Autodesk Fusion 360 part; units mm, degrees
sketch "Sketch1" plane through (0, 0, 0) normal (0, 1, 0) x (1, 0, 0)
  circle A0 centre (0, 0) radius 7.9
  dimension "d1" = 15.8
extrude "Extrude1" add sketch "Sketch1" against normal blind 5.5
sketch "Sketch2" plane through (0, -5.5, 0) normal (0, -1, 0) x (1, 0, 0)
  circle A0 centre (0, 0) radius 7.9
  circle A1 centre (0, 0) radius 3.5
  dimension "d4" = 7
extrude "Extrude2" add sketch "Sketch2" along normal blind 2.7 contours A1
fillet "Fillet1" radius 1.5 1 edges at (-3.2631, -8.2, -1.2657)
extrude "Extrude3" add 1 faces at (3.1441, 0, -2.759) along direction (0, 1, 0) blind 1.3 draft -73.5
sketch "Sketch3" plane through (0, 1.3, 0) normal (0, 1, 0) x (-1, 0, 0)
  circle A0 centre (0, 0) radius 3.5113
  circle A1 centre (0, 0) radius 1.6
  line L0 (-1.02, 1.2327) -> (-1.02, -1.2327)
  dimension "d11" = 3.2
  dimension "d12" = 1.02
extrude "Extrude4" cut sketch "Sketch3" against normal blind 9.3 contours A1 L0 picked at (-0.3273, 0.4001)
sketch "Sketch4" plane through (0, 0, 0) normal (1, 0, 0) x (0, 1, 0)
  line L0 (1.3, 0) -> (1.3, -3.5113)
  line L1 (1.3, 3.5113) -> (1.3, 0)
  line L2 (-8.2, 0) -> (-8.2, 2)
  line L3 (-8.2, -2) -> (-8.2, 0)
  line L4 (-5.5, -3.5) -> (-5.5, -7.9)
  line L5 (-5.5, 7.9) -> (-5.5, 3.5)
  line L6 (1.3, 3.5113) -> (0, 7.9)
  line L7 (1.3, -3.5113) -> (0, -7.9)
  arc A0 (-8.2, -2) -> (-6.7, -3.5) centre (-6.7, -2) ccw
  arc A1 (-6.7, 3.5) -> (-8.2, 2) centre (-6.7, 2) ccw
  line L8 (-5.5, 3.5) -> (-6.7, 3.5)
  line L9 (-5.5, -3.5) -> (-6.7, -3.5)
  line L10 (0, 7.9) -> (-5.5, 7.9)
  line L11 (0, -7.9) -> (-5.5, -7.9)
  line L12 (-5.5, 7.9) -> (-5.5, -7.9)
  line L13 (0, -7.9) -> (0, 7.9)
  circle A2 centre (-2.75, 9.2007) radius 2.5
  point P0 (-4.885, 7.9)
  point P1 (-0.615, 7.9)
  dimension "d15" = 0.615
  dimension "d16" = 0.615
  dimension "d17" = 5
revolve "Revolve1" cut sketch "Sketch4" angle 360 about axis through (0, 1.75, 0) along (0, 1, 0) contours L10 A2 picked at (-2.75, 7.5002)
For this review, take the finished solid that the model builds, in its own axes (mm). A direction names the side the tool comes from. Coordinates: 2 decimals unless noted, no trailing zeros. Order: outer loops, then holes, each group sorted by start corner. A loop starts at its lowest first (then second) coordinate and runs counter-clockwise, first axis right, second up. Notation, with made-up numbers: (50.25, 78.25) -> (66.25, 78.25) arc R11 cw to (66.25, 88.25) -> close; hole circle Ø7 at (-21.5, 57.5). An arc over 180 degrees is marked (long way). Return JSON: item names as keys, results as strings.
1. We need section A-A on x = 0. Write out the cut boundary in (y, z), and give its area (3 significant figures).
Answer block:
{"outline": "(-8.2, -2) arc R1.5 ccw to (-6.7, -3.5) -> (-5.5, -3.5) -> (-5.5, -7.9) -> (-4.88, -7.9) arc R2.5 cw to (-0.62, -7.9) -> (0, -7.9) -> (1.3, -3.51) -> (1.3, -1.6) -> (-8, -1.6) -> (-8, 1.6) -> (1.3, 1.6) -> (1.3, 3.51) -> (0, 7.9) -> (-0.62, 7.9) arc R2.5 cw to (-4.88, 7.9) -> (-5.5, 7.9) -> (-5.5, 3.5) -> (-6.7, 3.5) arc R1.5 ccw to (-8.2, 2) -> close", "area": "82.7 mm²"}
2. We need section D-D on y = -2. Write out the cut boundary in (x, z).
Answer block:
{"outline": "circle Ø13.63 at (0, 0); hole (1.02, -1.23) -> (1.02, 1.23) arc R1.6 ccw (long way) to start"}
3. We need section C-C on y = -1. Write out the cut boundary in (x, z), and give its area (3 significant figures).
Answer block:
{"outline": "circle Ø14.83 at (0, 0); hole (1.02, -1.23) -> (1.02, 1.23) arc R1.6 ccw (long way) to start", "area": "166 mm²"}
4. The part is to be moulded in two halves that separate along Z. For faces 4 (the cylindrical face through (-6.269, -5.188, 4.807)), 5 (the flat face through (1.02, -3, 0)), 6 (the flat face through (0, -8, 0)), 7 (the flat face through (3.4, -5.5, 1.6)), say which applies: +Z half, -Z half, draft (parallel to the pull), parting line (faces both ways), or undercut.
Answer block:
{"face 4": "parting line", "face 5": "undercut", "face 6": "undercut", "face 7": "draft"}
5. Machinability: for faces 1 (the cylindrical face through (3.233, -6.092, 1.341)), 2 (the cylindrical face through (-1.6, -3.28, -0.05)), 3 (the cylindrical face through (-6.269, -0.303, 4.807)), which of the approach directions +Z, -Z, +X, -X, +Y, -Y give a long, thin tool a straight path to every point of the face, cutting with its end or side? Answer none if there is none.
Answer block:
{"face 1": "-Y", "face 2": "+Y", "face 3": "+Y, -Y"}
6. We need section B-B on z = 0. Write out the cut boundary in (x, y).
Answer block:
{"outline": "(-7.9, -5.5) -> (-3.5, -5.5) -> (-3.5, -6.7) arc R1.5 ccw to (-2, -8.2) -> (2, -8.2) arc R1.5 ccw to (3.5, -6.7) -> (3.5, -5.5) -> (7.9, -5.5) -> (7.9, -4.88) arc R2.5 cw to (7.9, -0.62) -> (7.9, 0) -> (3.51, 1.3) -> (1.02, 1.3) -> (1.02, -8) -> (-1.6, -8) -> (-1.6, 1.3) -> (-3.51, 1.3) -> (-7.9, 0) -> (-7.9, -0.62) arc R2.5 cw to (-7.9, -4.88) -> close"}
7. For line 1 (X direction, y = -5.25, z = 0); line 2 (Z direction, x = 0.75, y = -6); line 3 (Z direction, x = 0, y = -4.75), list the stretches that pass through material, from the lowest coordinate up. Write a range as from..to.
Answer block:
{"line 1": "-7.9..-1.6, 1.02..7.9", "line 2": "-3.42..-1.41, 1.41..3.42", "line 3": "-7.7..-1.6, 1.6..7.7"}
8. For pin 1 Ø1.5 at (y, z) = (-3, 4.5) entering from -X; pin 2 Ø3 at (x, z) = (-1.5, -6.5) entering from +Y; pin 3 Ø1.3 at (x, z) = (-0.5, -0.5) entering from +Y, all flat-tipped, find the tip position at first contact; note any pin that passes through.
Answer block:
{"pin 1": "x = -5.59", "pin 2": "y = 0.81", "pin 3": "y = -8"}
